Print and shaded views of the part. All mm, measured from the part's lowest x, y and z. A direction names the side the tool comes from. Round coordinates to 2 decimals unless told otherwise and drop trailing zeros. Order: outer loops, then holes, each group sorted by start corner. A loop starts at its lowest first (then second) coordinate and runs counter-clockwise, first axis right, second up. Notation, with made-up numbers: (55.5, 64.25) - (70.5, 64.25) arc R31 cw to (70.5, 90.25) - close; hole circle Ø3 at (-7, -6). An arc over 180 degrees is marked (long way). Return JSON: item names as keys, results as strings. Group by question number.
Item 1: Saw through at A-A on z = 1.75. List the corners of the cut face in (x, y).
Item 2: Drop flat-ended pins along their axis: pin 1 (0.6 mm diameter, centred on y = 1.5, z = 1.5, fed in from +X); pin 2 (0.6 mm diameter, centred on y = 3.5, z = 1, fed in from -X). Give the stop position or say it passes through.
Item 3: Tool access for the marked faces 1, 2 and 3: list every direction of +Z, -Z, +X, -X, +Y, -Y with a clear straight run to the whole face (end or side of a thin tool).
Item 4: Two-plate mould, pull along X, no slides. Class the marked faces 4, 5, 6 and 7: released by +X, released by -X, zero draft, split by the parting line, or undercut.
Item 5: Saw through at B-B on y = 4.8. List the corners of the cut face in (x, z).
Item 6: Saw through at C-C on x = 5.75. List the corners of the cut face in (y, z).
Item 7: Probe probe 1 along Z at (x, y) = (7, 3.45); probe 2 along X at (y, z) = (1.85, 1.3); probe 3 along Z at (x, y) = (2, 1.9). List the from-to ranges inside material, lowest first.
Item 8: Saw through at D-D on x = 3. List the corners of the cut face in (y, z), and give its area (3 significant figures).
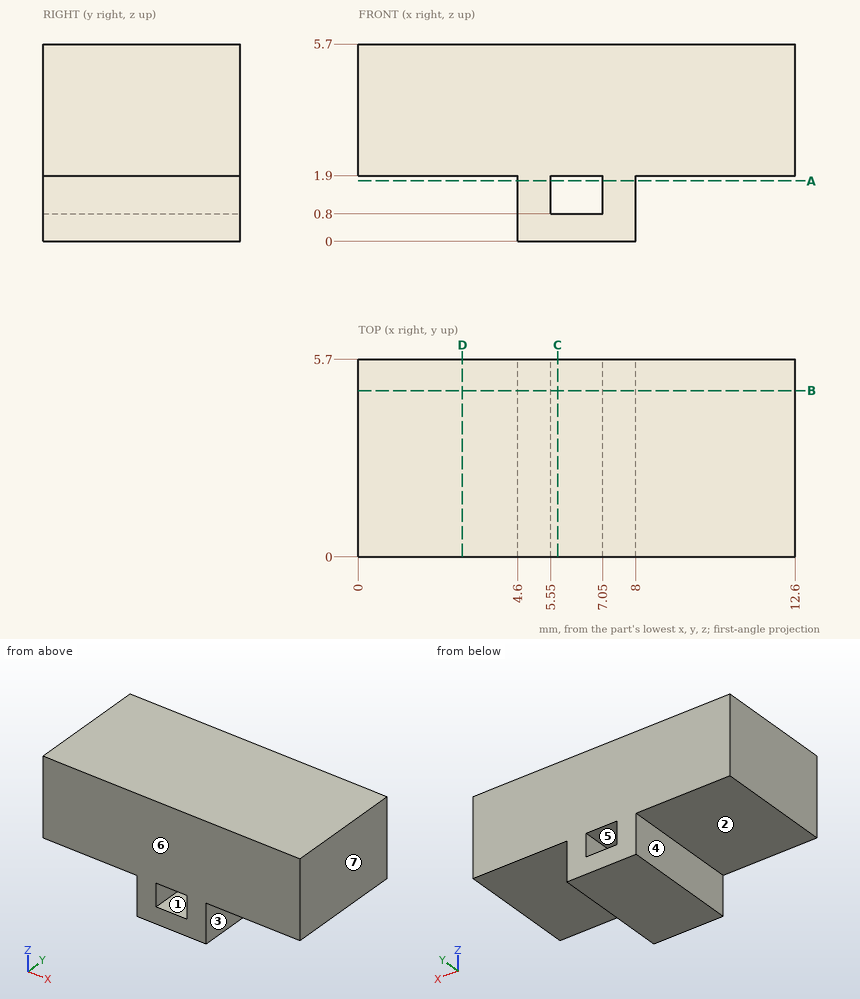
Filled in:
{
 "1": {"outline": "(4.6, 0) - (5.55, 0) - (5.55, 5.7) - (4.6, 5.7) - close; (7.05, 0) - (8, 0) - (8, 5.7) - (7.05, 5.7) - close"},
 "2": {"pin 1": "stops at x = 8", "pin 2": "stops at x = 4.6"},
 "3": {"face 1": "+Y, -Y", "face 2": "-Z, -X, +Y, -Y", "face 3": "-Z, +X, +Y, -Y"},
 "4": {"face 4": "released by -X", "face 5": "undercut", "face 6": "zero draft", "face 7": "released by +X"},
 "5": {"outline": "(0, 1.9) - (4.6, 1.9) - (4.6, 0) - (8, 0) - (8, 1.9) - (12.6, 1.9) - (12.6, 5.7) - (0, 5.7) - close; hole (5.55, 0.8) - (7.05, 0.8) - (7.05, 1.9) - (5.55, 1.9) - close"},
 "6": {"outline": "(0, 0) - (5.7, 0) - (5.7, 0.8) - (0, 0.8) - close; (0, 1.9) - (5.7, 1.9) - (5.7, 5.7) - (0, 5.7) - close"},
 "7": {"probe 1": "z = 0 to 0.8, 1.9 to 5.7", "probe 2": "x = 4.6 to 5.55, 7.05 to 8", "probe 3": "z = 1.9 to 5.7"},
 "8": {"outline": "(0, 1.9) - (5.7, 1.9) - (5.7, 5.7) - (0, 5.7) - close", "area": "21.7 mm^2"}
}
